Part model, mm, in its own coordinate system. A direction names the side the tool comes from. Give positions to 0.01 mm unless a question says otherwise; leave off trailing zeros. Write each loop counter-clockwise with the first axis right and the second up, starting at its lowest first coordinate (ties: lowest second). Pieces come first, ordered by that corner, then holes. Notation, with made-up numbers: M -11,73 L 2,73 A19 ccw 2,79 Z; hole C 54,-30 d3. An arc over 180 degrees is marked long. Use a Markdown table: item, result.
```python
from build123d import *

# Parameters (mm, degrees)
SKETCH_1_W          = 60
SKETCH_1_H          = 100
SKETCH_1_R          = 10
EXTRUDE_1_DEPTH     = 10
SKETCH_2_R          = 10
EXTRUDE_2_DEPTH     = 2
FILLET_1_R          = 20
SKETCH_3_W          = 60
SKETCH_3_H          = 50
EXTRUDE_3_DEPTH     = 5
SKETCH_4_R          = 2.25
CUT_EXTRUDE_1_DEPTH = 105.043260233


with BuildPart() as part:
    # 草图1 → 凸台-拉伸1 (new body)
    with BuildSketch(Plane.XY):
        with Locations((0, 50)):
            Rectangle(SKETCH_1_W, SKETCH_1_H)
        with Locations((0, 80)):
            Circle(SKETCH_1_R, mode=Mode.SUBTRACT)
    extrude(amount=EXTRUDE_1_DEPTH)

    # 草图2 → 凸台-拉伸2 (add)
    with BuildSketch(Plane(origin=(0, 0, 0), x_dir=(-1, 0, 0), z_dir=(0, 0, -1))):
        with Locations((0, 80)):
            Circle(SKETCH_2_R)
    extrude(amount=-EXTRUDE_2_DEPTH)

    # 圆角1
    fillet_1_edges = [part.edges().sort_by_distance(p)[0] for p in [
        (-30, 100, 5),
        (30, 100, 5),
    ]]
    fillet(fillet_1_edges, radius=FILLET_1_R)

    # 草图3 → 凸台-拉伸3 (add)
    with BuildSketch(Plane.XZ):
        with Locations((0, 5)):
            Rectangle(SKETCH_3_W, SKETCH_3_H)
    extrude(amount=-EXTRUDE_3_DEPTH)

    # 草图4 → 切除-拉伸1 (cut, through all)
    with BuildSketch(Plane(origin=(0, 5, 0), x_dir=(1, 0, 0), z_dir=(0, 1, 0))):
        with Locations(Location((-20, 10, 0), (0, 0, 270))):
            Circle(SKETCH_4_R)
        with Locations(Location((20, 10, 0), (0, 0, 270))):
            Circle(SKETCH_4_R)
        with Locations(Location((-20, -20, 0), (0, 0, 270))):
            Circle(SKETCH_4_R)
        with Locations(Location((20, -20, 0), (0, 0, 270))):
            Circle(SKETCH_4_R)
    extrude(amount=-CUT_EXTRUDE_1_DEPTH, mode=Mode.SUBTRACT)


solid = part.part
```
1. Cut at C-C, the plane x = 16. Give the cut face in (y, z), then the cut area to 3 significant figures.
Findings below:
| item | result |
|---|---|
| outline | M 0,-20 L 5,-20 L 5,0 L 99.08,0 L 99.08,10 L 5,10 L 5,30 L 0,30 Z |
| area | 1,190 mm2 |
2. Cut at A-A, the plane z = 20. Give the cut face in (x, y), then the cut area to 3 significant figures.
Findings below:
| item | result |
|---|---|
| outline | M -30,0 L -22.25,0 L -22.25,5 L -30,5 Z; M -17.75,0 L 17.75,0 L 17.75,5 L -17.75,5 Z; M 22.25,0 L 30,0 L 30,5 L 22.25,5 Z |
| area | 255 mm2 |
3. Drop flat-ended pins along their axis: P1, Ø10, axis at x = -6.5, z = -6, coming from the +Y side; P2, Ø12, axis at x = 5.5, y = 23, coming from the +Z side; P3, Ø2, axis at x = 11.5, y = 53, coming from the -Z side. Give the stop position or say it passes through.
Findings below:
| item | result |
|---|---|
| P1 | y = 5 |
| P2 | z = 10 |
| P3 | z = 0 |
4. Cut at B-B, the plane z = 4. Give the cut face in (x, y).
Findings below:
| item | result |
|---|---|
| outline | M -30,0 L 30,0 L 30,80 A20 ccw 10,100 L -10,100 A20 ccw -30,80 Z; hole C 0,80 d20 |
5. Tool access for faces 4 (the cylindrical face through (-23.986, 94.297, 5.07)), 5 (the flat face through (0, 53, 10)), 6 (the flat face through (0, 80, 2)), 7 (the flat face through (0, 53, 0)), 8 (the cylindrical face through (-21.996, 2.535, 21.038)): list every direction of +Z, -Z, +X, -X, +Y, -Y with a clear straight run to the whole face (end or side of a thin tool).
Findings below:
| item | result |
|---|---|
| face 4 | +Z, -Z, -X, +Y |
| face 5 | +Z, +X, -X, +Y |
| face 6 | +Z |
| face 7 | -Z, +X, -X, +Y |
| face 8 | +Y, -Y |
6. Two-plate mould, pull along X, no slides. Class faces 1 (the flat face through (0, 0, 5)), 2 (the flat face through (30, 31, 5)), 3 (the cylindrical face through (-1.302, 89.915, 5.944)): released by +X, released by -X, zero draft, split by the parting line, or undercut.
Findings below:
| item | result |
|---|---|
| face 1 | zero draft |
| face 2 | released by +X |
| face 3 | undercut |
7. Cut at D-D, the plane y = 22. Give the cut face in (x, z).
Findings below:
| item | result |
|---|---|
| outline | M -30,0 L 30,0 L 30,10 L -30,10 Z |
8. Drill centre lines: L1, parallel to X at y = 2.2, z = 20; L2, parallel to Y at x = 0, z = 7.5; L3, parallel to Z at x = -22.5, y = 23. Where is each one in solid material? Low to high.
Findings below:
| item | result |
|---|---|
| L1 | -30 to -22.25, -17.75 to 17.75, 22.25 to 30 |
| L2 | 0 to 70, 90 to 100 |
| L3 | 0 to 10 |
